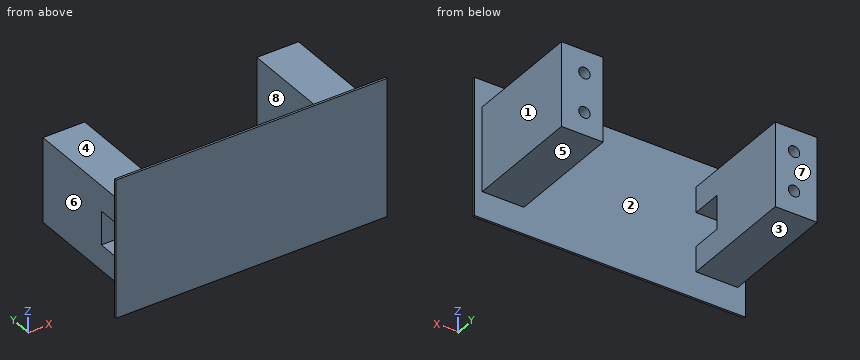
```python
from build123d import *

# Parameters (mm, degrees)
SKETCH1_W           = 65
SKETCH1_H           = 33
BOSS_EXTRUDE1_DEPTH = 0.5
SKETCH2_W           = 10
SKETCH2_H           = 20.24
BOSS_EXTRUDE2_DEPTH = 28.13
CUT_EXTRUDE1_START  = -10
SKETCH3_R           = 1.361077795
CUT_EXTRUDE1_DEPTH  = 57.348429315
CUT_EXTRUDE2_REACH  = 73.251
SKETCH4_W           = 8.1
SKETCH4_H           = 7.4


with BuildPart() as part:
    # Sketch1 → Boss-Extrude1 (new body)
    with BuildSketch(Plane(origin=(0, 0, 0), x_dir=(1, 0, 0), z_dir=(0, 1, 0))):
        Rectangle(SKETCH1_W, SKETCH1_H)
    extrude(amount=BOSS_EXTRUDE1_DEPTH)

    # Sketch2 → Boss-Extrude2 (add)
    with BuildSketch(Plane(origin=(0, 0.5, 0), x_dir=(1, 0, 0), z_dir=(0, 1, 0))):
        with Locations((25.625, 0)):
            Rectangle(SKETCH2_W, SKETCH2_H)
    boss_extrude2 = extrude(amount=BOSS_EXTRUDE2_DEPTH)

    # Sketch3 → Cut-Extrude1 (cut)
    with BuildSketch(Plane(origin=(0, 28.63, 0), x_dir=(1, 0, 0), z_dir=(0, 1, 0)).offset(CUT_EXTRUDE1_START)):
        with Locations(Location((25.125, 4.7, 0), (0, 0, 90))):
            Circle(SKETCH3_R)
        with Locations(Location((25.125, -4.7, 0), (0, 0, 90))):
            Circle(SKETCH3_R)
    cut_extrude1 = extrude(amount=CUT_EXTRUDE1_DEPTH, mode=Mode.SUBTRACT)

    # Mirror3: Boss-Extrude2, Cut-Extrude1 across plane
    add(boss_extrude2.mirror(Plane(origin=(0, 0, 0), x_dir=(0, 0, 1), z_dir=(1, 0, 0))))
    add(cut_extrude1.mirror(Plane(origin=(0, 0, 0), x_dir=(0, 0, 1), z_dir=(1, 0, 0))), mode=Mode.SUBTRACT)

    # Sketch4 → Cut-Extrude2 (cut, up to next)
    with BuildSketch(Plane.ZY.offset(30.625), mode=Mode.PRIVATE) as cut_extrude2_sk1:
        with Locations((0, 4.2)):
            Rectangle(SKETCH4_W, SKETCH4_H)
    cut_extrude2_tool1 = extrude(cut_extrude2_sk1.sketch, amount=-CUT_EXTRUDE2_REACH, mode=Mode.PRIVATE) & part.part
    add(cut_extrude2_tool1.solids().sort_by_distance((-30.625, 4.2, 0))[0], mode=Mode.SUBTRACT)


solid = part.part
```
Model file for the job. Use its own axes, mm. Face numbers are marked on the shaded views. A direction names the side the tool comes from. Coordinates: 2 decimals unless noted, no trailing zeros. Order: outer loops, then holes, each group sorted by start corner. A loop starts at its lowest first (then second) coordinate and runs counter-clockwise, first axis right, second up. Notation, with made-up numbers: (-36, 12) - (-8, 12) arc R18 cw to (-8, 28) - close; hole circle Ø10 at (79, -18.5). An arc over 180 degrees is marked (long way). Return JSON: item names as keys, results as strings. Group by question number.
1) Probe line 1 (X direction, y = 23, z = -4.7) (3 decimals); line 2 (X direction, y = 3.25, z = 8.5) (3 decimals); line 3 (X direction, y = 26, z = -5.5) (3 decimals). List the from-to ranges inside material, lowest first. Write a range as from..to.
2) Saw through at D-D, the plane y = 25.75. Write the cut outline in (x, z) (3 decimals).
3) Mould opens along X. For the marked faces 1, 2 and 3 say: released by +X, released by -X, zero draft, split by the parting line, or undercut.
4) Tool access for the marked faces 4, 5, 6, 7 and 8: list every direction of +Z, -Z, +X, -X, +Y, -Y with a clear straight run to the whole face (end or side of a thin tool).
5) Saw through at A-A, the plane y = 16. Write the cut outline in (x, z) (3 decimals).
6) Flat gauge pins, fed straight in: P1, Ø1.5, axis at x = 21.5, z = 12.5, coming from the +Y side; P2, Ø2, axis at x = -26.5, y = 2.5, coming from the +Z side; P3, Ø2.5, axis at x = 25.125, z = -4.7, coming from the +Y side. Where does each tip first touch, or does it go through?
7) Saw through at B-B, the plane z = -1. Write the cut outline in (x, y) (3 decimals).
8) Saw through at C-C, the plane y = 5.25. Write the cut outline in (x, z) (3 decimals).
Values found:
{
 "1": {"line 1": "x = -30.625..-26.486, -23.764..-20.625, 20.625..23.764, 26.486..30.625", "line 2": "x = -30.625..-20.625, 20.625..30.625", "line 3": "x = -30.625..-26.226, -24.024..-20.625, 20.625..24.024, 26.226..30.625"},
 "2": {"outline": "(-30.625, -10.12) - (-20.625, -10.12) - (-20.625, 10.12) - (-30.625, 10.12) - close; (20.625, -10.12) - (30.625, -10.12) - (30.625, 10.12) - (20.625, 10.12) - close; hole circle Ø2.722 at (-25.125, -4.7); hole circle Ø2.722 at (-25.125, 4.7); hole circle Ø2.722 at (25.125, -4.7); hole circle Ø2.722 at (25.125, 4.7)"},
 "3": {"face 1": "released by +X", "face 2": "undercut", "face 3": "zero draft"},
 "4": {"face 4": "+Z, +X, -X, +Y", "face 5": "-Z, +X, -X, +Y", "face 6": "+Z, -Z, -X, +Y", "face 7": "+Z, -Z, +X, -X, +Y", "face 8": "+Z, -Z, +Y"},
 "5": {"outline": "(-30.625, -10.12) - (-20.625, -10.12) - (-20.625, 10.12) - (-30.625, 10.12) - close; (20.625, -10.12) - (30.625, -10.12) - (30.625, 10.12) - (20.625, 10.12) - close"},
 "6": {"P1": "stops at y = 0.5", "P2": "stops at z = 10.12", "P3": "stops at y = 18.63"},
 "7": {"outline": "(-32.5, 0) - (32.5, 0) - (32.5, 0.5) - (30.625, 0.5) - (30.625, 28.63) - (20.625, 28.63) - (20.625, 0.5) - (-32.5, 0.5) - close; (-30.625, 7.9) - (-20.625, 7.9) - (-20.625, 28.63) - (-30.625, 28.63) - close"},
 "8": {"outline": "(-30.625, -10.12) - (-20.625, -10.12) - (-20.625, -4.05) - (-30.625, -4.05) - close; (-30.625, 4.05) - (-20.625, 4.05) - (-20.625, 10.12) - (-30.625, 10.12) - close; (20.625, -10.12) - (30.625, -10.12) - (30.625, 10.12) - (20.625, 10.12) - close"}
}
